from build123d import *

# Parameters (mm, degrees)
CROQUIS1_W              = 10
CROQUIS1_H              = 14
SALIENTE_EXTRUIR1_DEPTH = 4.5
CROQUIS2_W              = 8.2
CROQUIS2_H              = 4.08
CORTAR_EXTRUIR1_DEPTH   = 5
CORTAR_EXTRUIR2_REACH   = 19.455
CROQUIS3_W              = 5
CROQUIS3_H              = 3.66
CORTAR_EXTRUIR3_REACH   = 19.455
CROQUIS4_W              = 5
CROQUIS4_H              = 3.66
CORTAR_EXTRUIR4_REACH   = 19.783
CROQUIS5_W              = 2.5
CROQUIS5_H              = 0.8
CROQUIS6_W              = 2.5
CROQUIS6_H              = 0.8
CORTAR_EXTRUIR5_DEPTH   = 18.783419244
CORTAR_EXTRUIR6_REACH   = 15.01
CROQUIS7_W              = 2
CROQUIS7_H              = 0.8
CORTAR_EXTRUIR7_REACH   = 15.01
CROQUIS8_W              = 2
CROQUIS8_H              = 0.8


with BuildPart() as part:
    # Croquis1 → Saliente-Extruir1 (new body)
    with BuildSketch(Plane.XZ.offset(4.5)):
        with Locations((5, 0)):
            Rectangle(CROQUIS1_W, CROQUIS1_H)
    extrude(amount=-SALIENTE_EXTRUIR1_DEPTH)

    # Croquis2 → Cortar-Extruir1 (cut)
    with BuildSketch(Plane(origin=(10, 0, 0), x_dir=(0, 0, -1), z_dir=(1, 0, 0))):
        with Locations((0, -2.46)):
            Rectangle(CROQUIS2_W, CROQUIS2_H)
    extrude(amount=-CORTAR_EXTRUIR1_DEPTH, mode=Mode.SUBTRACT)

    # Croquis3 → Cortar-Extruir2 (cut, up to next)
    with BuildSketch(Plane.XY.offset(6.58), mode=Mode.PRIVATE) as cortar_extruir2_sk1:
        with Locations((7.5, -2.25)):
            Rectangle(CROQUIS3_W, CROQUIS3_H)
    cortar_extruir2_tool1 = extrude(cortar_extruir2_sk1.sketch, amount=-CORTAR_EXTRUIR2_REACH, mode=Mode.PRIVATE) & part.part
    add(cortar_extruir2_tool1.solids().sort_by_distance((7.5, -2.25, 6.58))[0], mode=Mode.SUBTRACT)

    # Croquis4 → Cortar-Extruir3 (cut, up to next)
    with BuildSketch(Plane(origin=(0, 0, -6.58), x_dir=(-1, 0, 0), z_dir=(0, 0, -1)), mode=Mode.PRIVATE) as cortar_extruir3_sk1:
        with Locations((-7.5, -2.25)):
            Rectangle(CROQUIS4_W, CROQUIS4_H)
    cortar_extruir3_tool1 = extrude(cortar_extruir3_sk1.sketch, amount=-CORTAR_EXTRUIR3_REACH, mode=Mode.PRIVATE) & part.part
    add(cortar_extruir3_tool1.solids().sort_by_distance((7.5, -2.25, -6.58))[0], mode=Mode.SUBTRACT)

    # Croquis5 → Cortar-Extruir4 (cut, up to next)
    with BuildSketch(Plane(origin=(0, 0, -7), x_dir=(-1, 0, 0), z_dir=(0, 0, -1)), mode=Mode.PRIVATE) as cortar_extruir4_sk1:
        with Locations((-8.75, -3.1)):
            Rectangle(CROQUIS5_W, CROQUIS5_H)
    cortar_extruir4_tool1 = extrude(cortar_extruir4_sk1.sketch, amount=-CORTAR_EXTRUIR4_REACH, mode=Mode.PRIVATE) & part.part
    add(cortar_extruir4_tool1.solids().sort_by_distance((8.75, -3.1, -7))[0], mode=Mode.SUBTRACT)

    # Croquis6 → Cortar-Extruir5 (cut, through all)
    with BuildSketch(Plane.XY.offset(7)):
        with Locations((8.75, -3.1)):
            Rectangle(CROQUIS6_W, CROQUIS6_H)
    extrude(amount=-CORTAR_EXTRUIR5_DEPTH, mode=Mode.SUBTRACT)

    # Croquis7 → Cortar-Extruir6 (cut, up to next)
    with BuildSketch(Plane.XZ.offset(4.5), mode=Mode.PRIVATE) as cortar_extruir6_sk1:
        with Locations((7.5, 5.55)):
            Rectangle(CROQUIS7_W, CROQUIS7_H)
    cortar_extruir6_tool1 = extrude(cortar_extruir6_sk1.sketch, amount=-CORTAR_EXTRUIR6_REACH, mode=Mode.PRIVATE) & part.part
    add(cortar_extruir6_tool1.solids().sort_by_distance((7.5, -4.5, 5.55))[0], mode=Mode.SUBTRACT)

    # Croquis8 → Cortar-Extruir7 (cut, up to next)
    with BuildSketch(Plane.XZ.offset(4.5), mode=Mode.PRIVATE) as cortar_extruir7_sk1:
        with Locations((7.5, -5.55)):
            Rectangle(CROQUIS8_W, CROQUIS8_H)
    cortar_extruir7_tool1 = extrude(cortar_extruir7_sk1.sketch, amount=-CORTAR_EXTRUIR7_REACH, mode=Mode.PRIVATE) & part.part
    add(cortar_extruir7_tool1.solids().sort_by_distance((7.5, -4.5, -5.55))[0], mode=Mode.SUBTRACT)


solid = part.part
CAD build for the part. Positions are in the model's coordinates, mm. A direction names the side the tool comes from. Give positions to 0.01 mm unless a question says otherwise; leave off trailing zeros. Write each loop counter-clockwise with the first axis right and the second up, starting at its lowest first coordinate (ties: lowest second). Pieces come first, ordered by that corner, then holes. Notation, with made-up numbers: (11.25, 17) - (16.25, 17) arc R35 cw to (16.25, 49) - close; hole circle Ø8 at (59, 24). An arc over 180 degrees is marked (long way). Answer as CSV lines item,"result".
Q1. Band-saw the part on C-C (y = -0.6). Give the cut face in (x, z).
Result set:
outline,"(0, -7) - (10, -7) - (10, -6.58) - (5, -6.58) - (5, 6.58) - (10, 6.58) - (10, 7) - (0, 7) - close"
Q2. 3-axis set-ups, long thin cutter, end or side, ignore diameter. For faces 4 (the face through (5, -2, 7)), 5 (the face through (8, -0.42, 0)): which of +Z, -Z, +X, -X, +Y, -Y reach the whole face in a straight line?
Result set:
face 4,"+Z, +X, -X, +Y, -Y"
face 5,"+X"
Q3. Band-saw the part on B-B (z = 3.75). Give the cut face in (x, y).
Result set:
outline,"(0, -4.5) - (5, -4.5) - (5, -0.42) - (10, -0.42) - (10, 0) - (0, 0) - close"
Q4. Band-saw the part on A-A (x = 9). Give the cut face in (y, z), and give its area (3 significant figures).
Result set:
outline,"(-4.5, -7) - (-3.5, -7) - (-3.5, -6.58) - (-4.08, -6.58) - (-4.08, -4.1) - (-4.5, -4.1) - close; (-4.5, 4.1) - (-4.08, 4.1) - (-4.08, 6.58) - (-3.5, 6.58) - (-3.5, 7) - (-4.5, 7) - close; (-2.7, -7) - (0, -7) - (0, 7) - (-2.7, 7) - (-2.7, 6.58) - (-0.42, 6.58) - (-0.42, -6.58) - (-2.7, -6.58) - close"
area,"10.7 mm²"
Q5. Flat gauge pins, fed straight in: pin 1 Ø0.5 at (x, z) = (8, 7) entering from +Y; pin 2 Ø1.5 at (x, z) = (6.5, -2.5) entering from -Y. Where does each tip first touch, or does it go through?
Result set:
pin 1,"y = 0"
pin 2,"y = -0.42"
Q6. Band-saw the part on D-D (x = 6.25). Give the cut face in (y, z), and give its area (3 significant figures).
Result set:
outline,"(-4.5, -7) - (0, -7) - (0, 7) - (-4.5, 7) - (-4.5, 4.1) - (-4.08, 4.1) - (-4.08, 6.58) - (-0.42, 6.58) - (-0.42, -6.58) - (-4.08, -6.58) - (-4.08, -4.1) - (-4.5, -4.1) - close"
area,"11.4 mm²"
Q7. Pull direction Y, two halves, no side cores. Call faces 1 (the face through (10, -4.23, 5.53)), 2 (the face through (7.5, -4.08, 4.8)), 3 (the face through (5, 0, 0)): released by +Y, released by -Y, zero draft, split by the parting line, or undercut.
Result set:
face 1,"zero draft"
face 2,"undercut"
face 3,"released by +Y"
Q8. Drill centre lines: line 1 (Z direction, x = 5.25, y = -2.2); line 2 (X direction, y = -2.35, z = -6.25); line 3 (Y direction, x = 5.5, z = 4.75). Where is each one in solid material? Low to high. Write a range as from..to.
Result set:
line 1,"-7..-6.58, 6.58..7"
line 2,"0..5"
line 3,"-4.5..-4.08, -0.42..0"
